from build123d import *

# Parameters (mm, degrees)
F1_DEPTH = 0.81


with BuildPart() as f1:
    # F0 (on Front) → F1 (new body)
    with BuildSketch(Plane.XZ):
        with BuildLine():
            Line((-6.475, 3.412853), (-6.475, 7.915))
            Line((-6.475, 7.915), (-14.605, 7.915))
            Line((-14.605, 7.915), (-14.605, -7.915))
            Line((-14.605, -7.915), (-14.605, -20.615))
            Line((-14.605, -20.615), (-6.475, -20.615))
            Line((-6.475, -20.615), (-6.475, -7.915))
            Line((-6.475, -7.915), (-0.638679, -7.915))
            ThreePointArc((-0.638679, -7.915), (2.770346, -6.092838), (3.149227, -2.245998))
            Line((3.149227, -2.245998), (1.127017, 2.636048))
            ThreePointArc((1.127017, 2.636048), (1.85222, 4.386842), (3.603014, 3.661639))
            Line((3.603014, 3.661639), (6.475, -3.271947))
            Line((6.475, -3.271947), (6.475, -7.915))
            Line((6.475, -7.915), (6.475, -20.615))
            Line((6.475, -20.615), (14.605, -20.615))
            Line((14.605, -20.615), (14.605, -7.915))
            Line((14.605, -7.915), (14.605, 7.915))
            Line((14.605, 7.915), (6.475, 7.915))
            Line((6.475, 7.915), (1.915, 7.915))
            ThreePointArc((1.915, 7.915), (-2.203111, 5.713824), (-2.6608, 1.066831))
            Line((-2.6608, 1.066831), (-1.13634, -2.613541))
            ThreePointArc((-1.13634, -2.613541), (-1.846951, -4.329109), (-3.562519, -3.618498))
            Line((-3.562519, -3.618498), (-6.475, 3.412853))
        make_face()
        with BuildLine():
            Line((-0.516458, -1.431615), (-1.377495, 0.647114))
            ThreePointArc((-1.377495, 0.647114), (-0.822769, 1.986341), (0.516458, 1.431615))
            Line((0.516458, 1.431615), (1.377495, -0.647114))
            ThreePointArc((1.377495, -0.647114), (0.822769, -1.986341), (-0.516458, -1.431615))
        make_face(mode=Mode.SUBTRACT)
    extrude(amount=F1_DEPTH)


solid = f1.part
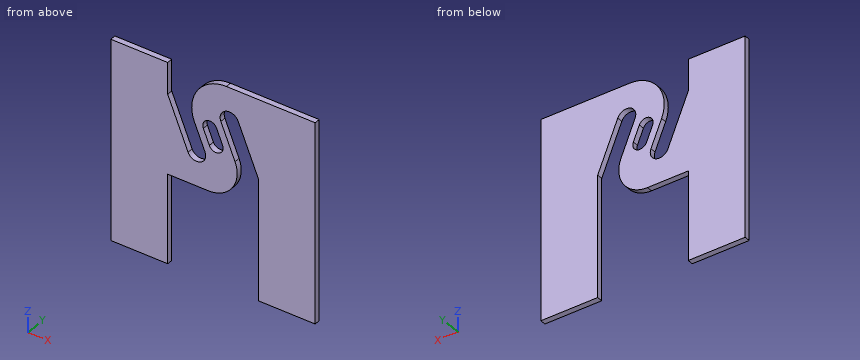
Verification items for the finished model (mm, model axes). Coordinates: 2 decimals unless noted, no trailing zeros. Loops run counter-clockwise (first coordinate to the right, second up) from the corner with the lowest first, then second, coordinate; pieces in that order, holes last. Notation, with made-up numbers: M 72,-29 L 80,-29 A22 ccw 80,6 Z; hole C 84.25,44.25 d1. An arc over 180 degrees is marked long. One line per item, written item: value.
1. Section check C-C on z = 0. Record the cut outline in (x, y) (3 decimals).
Answers follow:
outline: M -14.605,-0.81 L -5.061,-0.81 L -5.061,0 L -14.605,0 Z; M -2.219,-0.81 L -1.109,-0.81 L -1.109,0 L -2.219,0 Z; M 1.109,-0.81 L 2.219,-0.81 L 2.219,0 L 1.109,0 Z; M 5.12,-0.81 L 14.605,-0.81 L 14.605,0 L 5.12,0 Z
2. Section check A-A on z = -10.5. Record the cut outline in (x, y) (3 decimals).
Answers follow:
outline: M -14.605,-0.81 L -6.475,-0.81 L -6.475,0 L -14.605,0 Z; M 6.475,-0.81 L 14.605,-0.81 L 14.605,0 L 6.475,0 Z
3. Gauge pin test, flat end, axial feed: P1, Ø8, axis at x = -1.5, z = -16.5, coming from the -Y side. Record the tip position at first contact, or that the pin passes through.
Answers follow:
P1: through
4. Material ranges on line 1 along X through (y, z) = (-0.05, 2.5) (3 decimals); line 2 along X through (y, z) = (-0.3, -3.5) (3 decimals); line 3 along X through (y, z) = (-0.75, -9.75) (3 decimals), recorded low to high. Write a range as from..to.
Answers follow:
line 1: -14.605..-6.097, -3.016..1.183, 4.084..14.605
line 2: -14.605..-3.612, -1.094..3.449, 6.475..14.605
line 3: -14.605..-6.475, 6.475..14.605
5. Section check D-D on x = 5.5. Record the cut outline in (y, z) (3 decimals), plus the area to 3 significant figures.
Answers follow:
outline: M -0.81,-0.918 L 0,-0.918 L 0,7.915 L -0.81,7.915 Z
area: 7.15 mm^2
